```python
from build123d import *

# Parameters (mm, degrees)
BOSS_EXTRUDE1_DEPTH     = 9
CUT_EXTRUDE1_DEPTH      = 5.75
CUT_EXTRUDE1_DEPTH_BACK = 5.75
SKETCH3_R               = 2
CUT_EXTRUDE2_DEPTH      = 2
SKETCH4_R               = 1.5
CUT_EXTRUDE3_DEPTH      = 10


with BuildPart() as part:
    # Sketch1 → Boss-Extrude1 (new body)
    with BuildSketch(Plane(origin=(0, 0, 0), x_dir=(1, 0, 0), z_dir=(0, 1, 0))):
        with BuildLine():
            Line((-16.573076923, 2.982552816), (-0.511538462, 4.722375292))
            ThreePointArc((-0.511538462, 4.722375292), (4.75, 0), (-0.511538462, -4.722375292))
            Line((-0.511538462, -4.722375292), (-16.573076923, -2.982552816))
            ThreePointArc((-16.573076923, -2.982552816), (-19.25, 0), (-16.573076923, 2.982552816))
        make_face()
    extrude(amount=BOSS_EXTRUDE1_DEPTH)

    # Sketch2 → Cut-Extrude1 (cut, two sides)
    with BuildSketch(Plane.XY) as cut_extrude1_sk:
        Polygon((-4.75, 9), (-12.0546875, 6.25), (-19.25, 6.25), (-19.25, 9), align=None)
        Polygon((-13.25, 0), (-4.75, 3.2), (4.75, 3.2), (4.75, 0), align=None)
    extrude(amount=CUT_EXTRUDE1_DEPTH, mode=Mode.SUBTRACT)
    extrude(cut_extrude1_sk.sketch, amount=-CUT_EXTRUDE1_DEPTH_BACK, mode=Mode.SUBTRACT)

    # Sketch3 → Cut-Extrude2 (cut)
    with BuildSketch(Plane.XZ.offset(-3.2)):
        Circle(SKETCH3_R)
    extrude(amount=-CUT_EXTRUDE2_DEPTH, mode=Mode.SUBTRACT)

    # Sketch4 → Cut-Extrude3 (cut, through all)
    with BuildSketch(Plane.XZ):
        with Locations((-16.25, 0)):
            Circle(SKETCH4_R)
    extrude(amount=-CUT_EXTRUDE3_DEPTH, mode=Mode.SUBTRACT)


solid = part.part
```
Design review of the part built by this model. Coordinates are the model's own, in mm. A direction names the side the tool comes from. Give positions to 0.01 mm unless a question says otherwise; leave off trailing zeros. Loops run counter-clockwise (first coordinate to the right, second up) from the corner with the lowest first, then second, coordinate; pieces in that order, holes last. Notation, with made-up numbers: (44, -20) -> (88, -20) arc R22 cw to (88, 12) -> close; hole circle Ø6 at (73, 19.5). An arc over 180 degrees is marked (long way). Write each question's results on one line, items separated by ' | '.
Q1. For pin 1 Ø4 at (x, z) = (-12, 2.5) entering from +Y; pin 2 Ø1.2 at (x, z) = (0, 0.5) entering from -Y; pin 3 Ø3 at (x, z) = (-7, -2.5) entering from -Y, all flat-tipped, find the tip position at first contact; note any pin that passes through.
Reply:
pin 1: stops at y = 7.02 | pin 2: stops at y = 5.2 | pin 3: stops at y = 1.79
Q2. The part is to be moulded in two halves that separate along X. For faces 4 (the face through (-17.75, 3.08, 0.07)), 5 (the face through (-14, 0, 0)), 6 (the face through (-8.43, 4.437, 3.865)), say which applies: +X half, -X half, draft (parallel to the pull), parting line (faces both ways), or undercut.
Reply:
face 4: undercut | face 5: draft | face 6: -X half
Q3. Take a section at C-C, the plane y = 2.5. Write out the cut boundary in (x, z), plus the area to 3 significant figures.
Reply:
outline: (-16.57, -2.98) -> (-6.61, -4.06) -> (-6.61, 4.06) -> (-16.57, 2.98) arc R3 ccw to start; hole circle Ø3 at (-16.25, 0) | area: 75.3 mm²
Q4. Take a section at D-D, the plane x = 0. Write out the cut boundary in (y, z).
Reply:
outline: (3.2, -4.75) -> (9, -4.75) -> (9, 4.75) -> (3.2, 4.75) -> (3.2, 2) -> (5.2, 2) -> (5.2, -2) -> (3.2, -2) -> close
Q5. Take a section at B-B, the plane x = -16.25. Write out the cut boundary in (y, z), plus the area to 3 significant figures.
Reply:
outline: (0, -3.02) -> (6.25, -3.02) -> (6.25, -1.5) -> (0, -1.5) -> close; (0, 1.5) -> (6.25, 1.5) -> (6.25, 3.02) -> (0, 3.02) -> close | area: 19.0 mm²
Q6. Wall thickness on L1, parallel to Z at x = -17.25, y = 2; L2, parallel to Z at x = 0, y = 4.3; L3, parallel to Y at x = 2.5, z = -3.5: over which ranges is each line inside the solid? List them lowest first.
Reply:
L1: z = -2.83 to -1.12, 1.12 to 2.83 | L2: z = -4.75 to -2, 2 to 4.75 | L3: y = 3.2 to 9
Q7. Take a section at A-A, the plane z = 0. Write out the cut boundary in (x, y), plus the area to 3 significant figures.
Reply:
outline: (-19.25, 0) -> (-17.75, 0) -> (-17.75, 6.25) -> (-19.25, 6.25) -> close; (-14.75, 0) -> (-13.25, 0) -> (-4.75, 3.2) -> (-2, 3.2) -> (-2, 5.2) -> (2, 5.2) -> (2, 3.2) -> (4.75, 3.2) -> (4.75, 9) -> (-4.75, 9) -> (-12.05, 6.25) -> (-14.75, 6.25) -> close | area: 115 mm²
Q8. Machinability: for faces 1 (the face through (0, 5.2, 0)), 2 (the face through (-2.2, 3.2, 0.1)), 3 (the face through (-14.8, 6.25, 0.8)), which of the approach directions +Z, -Z, +X, -X, +Y, -Y give a long, thin tool a straight path to every point of the face, cutting with its end or side? Answer none if there is none.
Reply:
face 1: -Y | face 2: +Z, -Z, +X, -Y | face 3: +Z, -Z, -X, +Y
